Autodesk Inventor part; units mm, degrees
ref_plane "YZ Plane" through (0, 0, 0) normal (1, 0, 0) x (0, 1, 0)
ref_plane "XZ Plane" through (0, 0, 0) normal (0, 1, 0) x (-1, 0, 0)
ref_plane "XY Plane" through (0, 0, 0) normal (0, 0, 1) x (1, 0, 0)
sketch "Sketch1" plane through (0, 0, 0) normal (0, 0, 1) x (1, 0, 0)
  line L0 (0, 0) -> (80, 0)
  circle A0 centre (0, 0) radius 5
  arc A1 (-3.75, 9.2702) -> (-3.75, -9.2702) centre (0, 0) ccw
  circle A2 centre (80, 0) radius 5
  arc A3 (83.75, -9.2702) -> (83.75, 9.2702) centre (80, 0) ccw
  circle A4 centre (40, 0) radius 12.5
  line L1 (-3.75, 9.2702) -> (30.625, 23.1756)
  line L2 (-3.75, -9.2702) -> (30.625, -23.1756)
  line L3 (49.375, -23.1756) -> (83.75, -9.2702)
  line L4 (106.6667, 0) -> (111.5084, 1.9586)
  line L5 (49.375, 23.1756) -> (83.75, 9.2702)
  line L6 (106.6667, 0) -> (112.4269, -2.3301)
  arc A5 (30.625, -23.1756) -> (49.375, -23.1756) centre (40, 0) ccw
  arc A6 (49.375, 23.1756) -> (30.625, 23.1756) centre (40, 0) ccw
  dimension "d0" = 80
  dimension "d1" = 20
  dimension "d2" = 10
  dimension "d4" = 25
  dimension "d5" = 20
  dimension "d6" = 10
  dimension "d7" = 40
extrude "Extrusion1" add sketch "Sketch1" along normal mid plane 15
Verification items for the finished model (mm, model axes). Give positions to 0.01 mm unless a question says otherwise; leave off trailing zeros. Write each loop counter-clockwise with the first axis right and the second up, starting at its lowest first coordinate (ties: lowest second). Pieces come first, ordered by that corner, then holes. Notation, with made-up numbers: M 84,74.25 L 121,74.25 A29 ccw 121,99.25 Z; hole C 88.5,84.5 d10. An arc over 180 degrees is marked long. One line per question, with ' | ' between items.
1) Section check B-B on z = -0.5. Enter the section's corners in (x, y) (3 decimals), plus the area to 3 significant figures.
Result:
outline: M -3.75,-9.27 L 30.625,-23.176 A25 ccw 49.375,-23.176 L 83.75,-9.27 A10 ccw 83.75,9.27 L 49.375,23.176 A25 ccw 30.625,23.176 L -3.75,9.27 A10 ccw Z; hole C 0,0 d10; hole C 40,0 d25; hole C 80,0 d10 | area: 2,670 mm2
2) Section check D-D on y = 7. Enter the section's corners in (x, z), plus the area to 3 significant figures.
Result:
outline: M -7.14,-7.5 L 29.64,-7.5 L 29.64,7.5 L -7.14,7.5 Z; M 50.36,-7.5 L 87.14,-7.5 L 87.14,7.5 L 50.36,7.5 Z | area: 1,100 mm2
3) Gauge pin test, flat ends, axial feed: pin 1 Ø2 at (y, z) = (18, -2) entering from -X; pin 2 Ø9 at (x, y) = (80, 0) entering from +Z; pin 3 Ø2 at (y, z) = (-17.5, 0) entering from +X; pin 4 Ø1.5 at (y, z) = (8.5, -4.5) entering from -X. Record the tip position at first contact, or that the pin passes through.
Result:
pin 1: stops at x = 15.36 | pin 2: passes through | pin 3: stops at x = 65.88 | pin 4: stops at x = -6.32
4) Section check A-A on x = 40. Enter the section's corners in (y, z).
Result:
outline: M -25,-7.5 L -12.5,-7.5 L -12.5,7.5 L -25,7.5 Z; M 12.5,-7.5 L 25,-7.5 L 25,7.5 L 12.5,7.5 Z
5) Mould release check, pull along X, two halves, no side actions. Record for faces 1 (the cylindrical face through (27.512, -0.55, -0.105)), 2 (the flat face through (66.32, 16.32, -0.11)), 3 (the cylindrical face through (40, 25, 0)), 4 (the cylindrical face through (84.619, 1.915, -0.105)): released by +X, released by -X, zero draft, split by the parting line, or undercut.
Result:
face 1: undercut | face 2: released by +X | face 3: split by the parting line | face 4: undercut
6) Thickness scan on line 1 along X through (y, z) = (-1, -6.5); line 2 along Y through (x, z) = (0, -4); line 3 along Y through (x, z) = (4, 4). Record the ranges inside material, lowest first. Write a range as [from, to].
Result:
line 1: x = [-9.95, -4.9], [4.9, 27.54], [52.46, 75.1], [84.9, 89.95] | line 2: y = [-10.79, -5], [5, 10.79] | line 3: y = [-12.41, -3], [3, 12.41]
7) Section check C-C on y = 0. Enter the section's corners in (x, z).
Result:
outline: M -10,-7.5 L -5,-7.5 L -5,7.5 L -10,7.5 Z; M 5,-7.5 L 27.5,-7.5 L 27.5,7.5 L 5,7.5 Z; M 52.5,-7.5 L 75,-7.5 L 75,7.5 L 52.5,7.5 Z; M 85,-7.5 L 90,-7.5 L 90,7.5 L 85,7.5 Z
